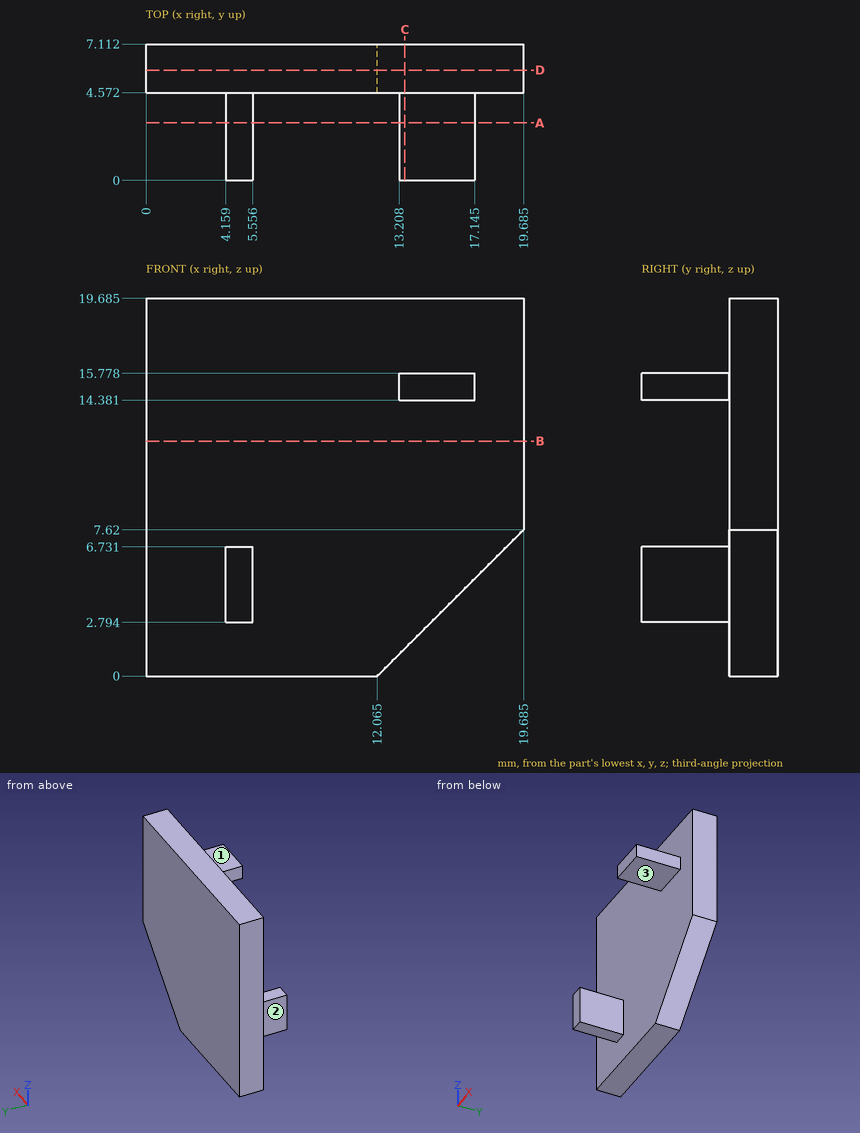
Drawing for the job (mm, zero at the part's lowest x, y, z). A direction names the side the tool comes from. Coordinates: 2 decimals unless noted, no trailing zeros. Order: outer loops, then holes, each group sorted by start corner. A loop starts at its lowest first (then second) coordinate and runs counter-clockwise, first axis right, second up. Notation, with made-up numbers: (14, -19) - (24, -19) arc R23 ccw to (24, 11) - close; hole circle Ø1 at (-9, 68). An arc over 180 degrees is marked (long way). Use a Markdown table: item, result. Add a question column.
(1) Saw through at C-C (x = 13.5). Give the cut face in (y, z) (1 decimal).
(2) Saw through at D-D (y = 5.75). Give the cut face in (x, z) (1 decimal).
(3) Which spindle directions (+Z, -Z, +X, -X, +Y, -Y) get a long thin tool onto all of the face, cutting with end or side? Do the marked faces 1, 2 and 3. Say none if no direction does.
(4) Saw through at B-B (z = 12.25). Give the cut face in (x, y) (1 decimal), then the cut area to 3 significant figures.
(5) Drill centre lines: line 1 along Z through (x, y) = (4.25, 4.5); line 2 along Y through (x, z) = (17.5, 15.75); line 3 along X through (y, z) = (1, 4). Where is each one in solid material? Low to high. Write a range as [from, to].
(6) Saw through at A-A (y = 3). Give the cut face in (x, z) (1 decimal), then the cut area to 3 significant figures.
(7) Flat gauge pins, fed straight in: pin 1 (1.5 mm diameter, centred on y = 1.5, z = 15.5, fed in from -X); pin 2 (0.7 mm diameter, centred on x = 5, y = 3, fed in from +Z); pin 3 (1 mm diameter, centred on x = 3, z = 6, fed in from -Y). Where does each tip first touch, or does it go through?
Solved:
| question | item | result |
|---|---|---|
| 1 | outline | (0, 14.4) - (4.6, 14.4) - (4.6, 1.4) - (7.1, 1.4) - (7.1, 19.7) - (4.6, 19.7) - (4.6, 15.8) - (0, 15.8) - close |
| 2 | outline | (0, 0) - (12.1, 0) - (19.7, 7.6) - (19.7, 19.7) - (0, 19.7) - close |
| 3 | face 1 | +Z, +X, -X, -Y |
| 3 | face 2 | +Z, -Z, -X, -Y |
| 3 | face 3 | -Z, +X, -X, -Y |
| 4 | outline | (0, 4.6) - (19.7, 4.6) - (19.7, 7.1) - (0, 7.1) - close |
| 4 | area | 50.0 mm² |
| 5 | line 1 | z = [2.79, 6.73] |
| 5 | line 2 | y = [4.57, 7.11] |
| 5 | line 3 | x = [4.16, 5.56] |
| 6 | outline | (4.2, 2.8) - (5.6, 2.8) - (5.6, 6.7) - (4.2, 6.7) - close; (13.2, 14.4) - (17.1, 14.4) - (17.1, 15.8) - (13.2, 15.8) - close |
| 6 | area | 11.0 mm² |
| 7 | pin 1 | stops at x = 13.21 |
| 7 | pin 2 | stops at z = 6.73 |
| 7 | pin 3 | stops at y = 4.57 |
